Can you work these out from the model? Positions are in its coordinate system, mm. Give positions to 0.01 mm unless a question says otherwise; leave off trailing zeros. Order: outer loops, then holes, each group sorted by start corner. A loop starts at its lowest first (then second) coordinate and runs counter-clockwise, first axis right, second up.
Item 1: I want a section at A-A, the plane y = 15. Write out the boundary of the cut face in (x, z).
Item 2: I'm going to push flat-ended pins straight in: pin 1 Ø0.7 at (x, y) = (3.5, 21) entering from +Z; pin 2 Ø11 at (y, z) = (7.5, -33) entering from +X; pin 3 Ø3 at (x, y) = (-28, -10.5) entering from +Z. Where does each tip first touch, or does it pass through?
Item 3: If I drill on line 1 along Y through (x, z) = (3.5, -66.5); line 2 along X through (y, z) = (14, -65); line 3 along Z through (x, y) = (1, 14.5), over which ranges is the centre line in solid material (lowest first)?
Item 4: I want a section at B-B, the plane z = -42. Write out the boundary of the cut face in (x, y), then the cut area to 3 significant figures.
Item 5: I want a section at C-C, the plane x = -21. Write out the boundary of the cut face in (y, z), then the cut area to 3 significant figures.
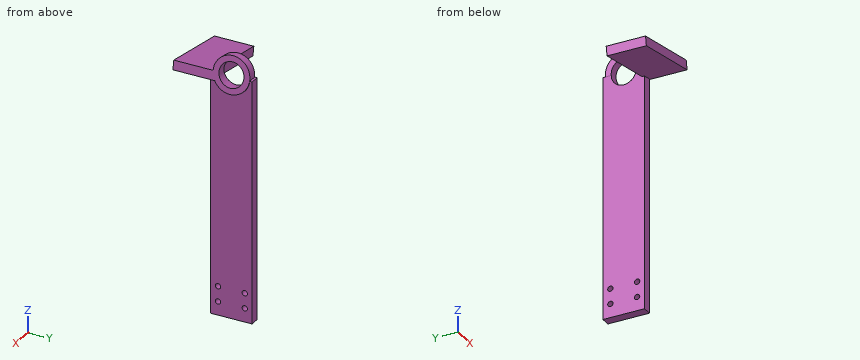
Autodesk Inventor part; units mm, degrees
ref_plane "YZ Plane" through (0, 0, 0) normal (1, 0, 0) x (0, 1, 0)
ref_plane "XZ Plane" through (0, 0, 0) normal (0, 1, 0) x (-1, 0, 0)
ref_plane "XY Plane" through (0, 0, 0) normal (0, 0, 1) x (1, 0, 0)
sketch "Sketch1" plane through (0, 0, 0) normal (1, 0, 0) x (0, 1, 0)
  line L0 (0, 0) -> (21.59, 0)
  line L1 (21.59, 0) -> (21.59, -127)
  line L2 (21.59, -127) -> (0, -127)
  line L3 (0, -127) -> (0, 0)
  dimension "d0" = 21.59
  dimension "d1" = 127
extrude "Extrusion1" add sketch "Sketch1" along normal blind 4.7625
sketch "Sketch2" plane through (0, 21.59, 0) normal (0, 1, 0) x (1, 0, 0)
  line L0 (0, 0) -> (-3.2071, -18.1884)
  line L1 (0, 0) -> (18.469, 0) construction
  line L2 (0, 0) -> (13.0579, -2.3025)
  line L3 (0, 0) -> (13.2594, 0) construction
  dimension "d4" = 100
  dimension "d24" = 10
ref_plane "Work Plane1" through (0, 21.59, 0) normal (-0.9848078, 0, -0.1736482) x (-0.1736482, 0, 0.9848078)
sketch "Sketch3" plane through (0, 21.59, 0) normal (-0.9848078, 0, -0.1736482) x (-0.1736482, 0, 0.9848078)
  line L0 (-0.827, 0) -> (-0.827, -21.59)
  line L1 (-0.827, -21.59) -> (-125.8976, -21.59)
  line L2 (-125.8976, -21.59) -> (-125.8976, 0)
  line L3 (-125.8976, 0) -> (-0.827, 0)
  line L4 (0, -21.59) -> (0, 0)
  line L5 (0, -21.59) -> (-0.827, -21.59)
  line L6 (-0.827, 0) -> (-0.827, -21.59)
  line L7 (0, 0) -> (-0.827, 0)
  line L8 (0, -21.59) -> (0, 0)
  circle A0 centre (0, -10.795) radius 9.525
  dimension "d5" = 19.05
  dimension "d6" = 21.59
  dimension "d7" = 10.795
extrude "Extrusion2" add sketch "Sketch3" against normal blind 4.7625 contours A0 L4 L0 | L0 A0 | A0 L4
sketch "Sketch5" plane through (4.6901, 10.795, 0.827) normal (0.9848078, 0, 0.1736482) x (0.1736482, 0, -0.9848078)
  circle A0 centre (0, 0) radius 9.525
  point P0 (0, -10.795)
hole "Hole2" at (4.6901, 10.795, 0.827) direction (-0.9848078, 0, -0.1736482) diameter 12.954 end through all
ref_plane "Work Plane3" through (0, 0, 0) normal (-0.1736482, 0, 0.9848078) x (0, 1, 0)
sketch "Sketch9" plane through (4.7625, 0, 0) normal (1, 0, 0) x (0, 0, -1)
  line L0 (0, 0) -> (127, 0)
  line L1 (127, 0) -> (127, 21.59)
  line L2 (127, 21.59) -> (0, 21.59)
  line L3 (0, 21.59) -> (0, 20.284)
  ellipse E0 centre (-0.8398, 10.795) end of major axis (8.8322, 10.795) minor radius 9.525 (0, 1.306) -> (0, 20.284) ccw
  circle A0 centre (115.825, 10.795) radius 8
  line L4 (111.825, 17.7232) -> (119.825, 17.7232)
  line L5 (119.825, 17.7232) -> (119.825, 3.8668)
  line L6 (119.825, 3.8668) -> (111.825, 3.8668)
  line L7 (111.825, 3.8668) -> (111.825, 17.7232)
  line L8 (0, 1.306) -> (0, 0)
  dimension "d34" = 16
  dimension "d35" = 8
  dimension "d36" = 4
  dimension "d37" = 21.59
  dimension "d38" = 10.795
  dimension "d39" = 11.175
hole "Hole3" at (4.7625, 17.7232, -111.825) at (4.7625, 17.7232, -119.825) at (4.7625, 3.8668, -119.825) at (4.7625, 3.8668, -111.825) direction (-1, 0, 0) diameter 2.794 end through all
sketch "Sketch10" plane through (0, 0, 0) normal (-0.1736482, 0, 0.9848078) x (0, 1, 0)
  ellipse E0 centre (10.795, 0) end of major axis (10.795, -54.019) minor radius 9.525 (20.284, -4.6901) -> (1.27, 0) ccw
  line L0 (1.27, 0) -> (20.32, 0)
  ellipse E1 centre (10.795, 0) end of major axis (10.795, -54.019) minor radius 9.525 (20.32, 0) -> (1.306, -4.6901) ccw
  ellipse E2 centre (10.795, -4.836) end of major axis (1.27, -4.836) minor radius 1.6795 (20.284, -4.6901) -> (1.306, -4.6901) ccw
  line L1 (1.27, -4.7625) -> (20.32, -4.7625)
  ellipse E3 centre (3.8668, 20.8074) end of major axis (5.2638, 20.8074) minor radius 0.2426
  ellipse E4 centre (17.7232, 19.4182) end of major axis (19.1202, 19.4182) minor radius 0.2426
  ellipse E5 centre (17.7232, 20.8074) end of major axis (19.1202, 20.8074) minor radius 0.2426
  ellipse E6 centre (3.8668, 19.4182) end of major axis (5.2638, 19.4182) minor radius 0.2426
  ellipse E7 centre (10.795, 0) end of major axis (17.272, 0) minor radius 1.1421 (17.272, 0) -> (4.318, 0) ccw
  line L2 (17.272, 0) -> (20.32, 0)
  line L3 (20.32, 0) -> (21.59, 0)
  line L4 (21.59, 0) -> (21.59, 22.0533)
  line L5 (21.59, 22.0533) -> (0, 22.0533)
  line L6 (0, 22.0533) -> (0, 0)
  line L7 (0, 0) -> (1.27, 0)
  line L8 (1.27, 0) -> (4.318, 0)
  line L9 (20.32, 0) -> (1.27, 0)
  line L10 (3.0923, 0) -> (1.27, 0)
  line L11 (-19.1327, 0) -> (-19.1327, -4.7625)
  line L12 (-19.1327, -4.7625) -> (3.0923, -4.7625)
  line L13 (3.0923, -4.7625) -> (3.0923, 0)
  line L14 (-19.1327, -4.7625) -> (1.27, -4.7625)
  line L15 (1.27, 0) -> (1.27, 35.6235)
  line L16 (1.27, 35.6235) -> (-19.1327, 35.6235)
  line L17 (-19.1327, 35.6235) -> (-19.1327, -4.7625)
  dimension "d47" = 22.225
  dimension "d50" = 20.4027
  dimension "d53" = 4.7625
  dimension "d54" = 40.386
extrude "Extrusion4" add sketch "Sketch10" against normal blind 4.7625 contours L13 L1 L12 L11 L17 L16 L15 L5 L6 L7 E1 E2 | E2 E1 L0 L13 | L7 L6 L5 L15
equation "\"d7\" = 0.5 * d6"
equation "\"d36\" = 0.5 * d35"
equation "\"d38\" = 0.5 * d37"
properties part number "WheelIntakeMotorMount2.0"
Results list:
1. outline: (-1.48, 8.42) - (-0.86, 4.85) - (3.83, 5.68) - (3.21, 9.24) - close; (0, -127) - (4.76, -127) - (4.76, -7.84) - (6.17, -7.59) - (5.55, -4.02) - (0, -5) - close
2. pin 1: stops at z = 0
2. pin 2: stops at x = 4.76
2. pin 3: stops at z = -4.67
3. line 1: y = 0 to 21.59
3. line 2: x = 0 to 4.76
3. line 3: z = -127 to -5.22, 5.57 to 9.09
4. outline: (0, 0) - (4.76, 0) - (4.76, 21.59) - (0, 21.59) - close
4. area: 103 mm2
5. outline: (-19.13, -8.54) - (1.27, -8.54) - (1.27, -3.7) - (-19.13, -3.7) - close
5. area: 98.7 mm2
